Autodesk Inventor part; units mm, degrees
ref_plane "YZ Plane" through (0, 0, 0) normal (1, 0, 0) x (0, 1, 0)
ref_plane "XZ Plane" through (0, 0, 0) normal (0, 1, 0) x (-1, 0, 0)
ref_plane "XY Plane" through (0, 0, 0) normal (0, 0, 1) x (1, 0, 0)
sketch "Sketch2" plane through (0, 0, 0) normal (0, 0, 1) x (1, 0, 0)
  line L0 (99.6671, 2.919) -> (99.6671, -3.431)
  line L1 (99.6671, -3.431) -> (-13.8455, -3.431)
  line L2 (-13.8455, -3.431) -> (-13.8455, 2.919)
  line L3 (-9.8831, 2.919) -> (-9.8831, 9.269)
  line L4 (-9.8831, 9.269) -> (-13.8455, 9.269)
  line L5 (-13.8455, 9.269) -> (-13.8455, 2.919)
  line L6 (-9.8831, 2.919) -> (99.6671, 2.919)
  line L7 (-13.8455, 11.6503) -> (99.6671, 11.6503)
  point P0 (0, 0)
  dimension "d17" = 113.5126
  dimension "d18" = 6.35
  dimension "d19" = 3.9624
  dimension "d20" = 6.35
  dimension "d24" = 6.35
  dimension "d25" = 6.35
  dimension "d26" = 113.5126
  dimension "d27" = 2.3813
revolve "Revolution1" add sketch "Sketch2" angle 360 about axis through (-13.8455, 11.6503, 0) along (1, 0, 0)
fillet "Fillet3" radius 6.35 2 edges at (99.6671, 26.7315, 0) (-13.8455, 26.7315, 0)
properties part number "rubberhandlesleeve"
Source: CAD feature listing. Evaluate the final solid. Frame: model axes, mm. Give positions to 0.01 mm unless a question says otherwise; leave off trailing zeros. Write each loop counter-clockwise with the first axis right and the second up, starting at its lowest first coordinate (ties: lowest second). Pieces come first, ordered by that corner, then holes. Notation, with made-up numbers: (77, 0.25) -> (109, 0.25) arc R15 cw to (109, 8.25) -> close; hole circle Ø10 at (87.25, 88). An arc over 180 degrees is marked (long way). Return JSON: item names as keys, results as strings. Group by question number.
1. Material intervals for line 1 (Z direction, x = 80.5, y = 11.5); line 2 (X direction, y = 6.5, z = 0); line 3 (Y direction, x = 57, z = 0), sorted ascending. Write a range as from..to.
2. Mould query, pull axis Y, two halves, no side actions, for faces 1 (the face through (-9.883, 10, 2)), 2 (the face through (-11.89, 14.03, 0.1)), 3 (the face through (42.2, 23.6, -9.2)), 4 (the face through (-13.846, 10, 2)). Classes: +Y half, -Y half, draft (parallel to the pull), parting line (faces both ways), or undercut.
3. Pin query (flat end, axial travel): pin 1 Ø1 at (x, z) = (25.5, -6) entering from -Y; pin 2 Ø2 at (y, z) = (10, 2) entering from +X; pin 3 Ø3 at (x, y) = (23.5, 6.5) entering from -Z; pin 4 Ø10 at (x, y) = (36, 12) entering from +Z. Return the tip coordinate at first contact, or that it passes through.
4. Section B-B, the plane x = -5.5. Output: boundary loops of the cut face in (y, z).
Determined:
{
 "1": {"line 1": "z = -15.08..-8.73, 8.73..15.08", "line 2": "x = -13.85..-9.88", "line 3": "y = -3.43..2.92, 20.38..26.73"},
 "2": {"face 1": "undercut", "face 2": "undercut", "face 3": "parting line", "face 4": "draft"},
 "3": {"pin 1": "stops at y = -2.39", "pin 2": "stops at x = -9.88", "pin 3": "stops at z = -14.63", "pin 4": "stops at z = 15.08"},
 "4": {"outline": "circle Ø30.16 at (11.65, 0); hole circle Ø17.46 at (11.65, 0)"}
}
